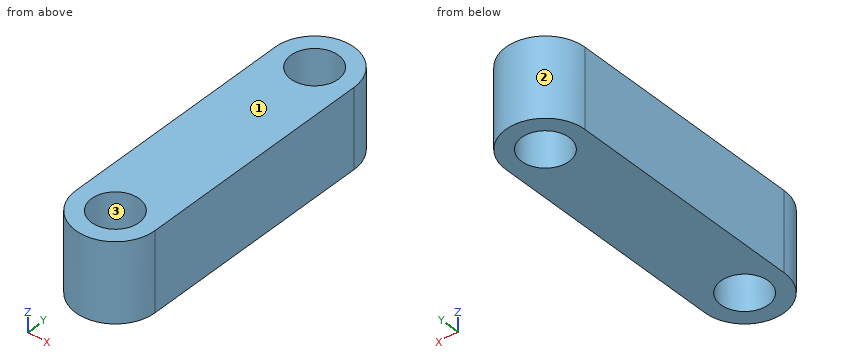
Autodesk Inventor part; units mm, degrees
ref_plane "YZ Plane" through (0, 0, 0) normal (1, 0, 0) x (0, 1, 0)
ref_plane "XZ Plane" through (0, 0, 0) normal (0, 1, 0) x (-1, 0, 0)
ref_plane "XY Plane" through (0, 0, 0) normal (0, 0, 1) x (1, 0, 0)
sketch "Sketch1" plane through (0, 0, 0) normal (0, 0, 1) x (1, 0, 0)
  circle A0 centre (0, 0) radius 1.5
  circle A1 centre (0, 0) radius 2.5
  line L0 (0, 0) -> (0, 15)
  circle A2 centre (0, 15) radius 1.5
  circle A3 centre (0, 15) radius 2.5
  line L1 (-2.5, 0) -> (-2.5, 15)
  line L2 (2.5, 0) -> (2.5, 15)
  dimension "d0" = 3
  dimension "d1" = 5
  dimension "d2" = 15
  dimension "d3" = 3
  dimension "d4" = 5
extrude "Extrusion1" add sketch "Sketch1" along normal blind 5
properties part number "bar_mid_2"
Verification items for the finished model (mm, model axes). Face numbers are marked on the shaded views. Round coordinates to 2 decimals unless told otherwise and drop trailing zeros. Order: outer loops, then holes, each group sorted by start corner. A loop starts at its lowest first (then second) coordinate and runs counter-clockwise, first axis right, second up. Notation, with made-up numbers: (52.25, 21.5) -> (80.25, 21.5) arc R21 ccw to (80.25, 58.5) -> close; hole circle Ø7 at (0.5, -1.75). An arc over 180 degrees is marked (long way). Put each result on its own line as item: value.
1) Depth check by flat-ended pin: pin 1 (1.8 mm diameter, centred on x = 0, y = 15, fed in from +Z). Enter the tip coordinate at first touch or a pass-through.
Final values:
pin 1: passes through
2) Section check C-C (y = 15.25). Record the cut outline in (x, z), then the cut area to 3 significant figures.
Final values:
outline: (-2.49, 0) -> (-1.48, 0) -> (-1.48, 5) -> (-2.49, 5) -> close; (1.48, 0) -> (2.49, 0) -> (2.49, 5) -> (1.48, 5) -> close
area: 10.1 mm^2
3) Mould release check, pull along X, two halves, no side actions. Record for the marked faces 1, 2 and 3: +X half, -X half, draft (parallel to the pull), parting line (faces both ways), or undercut.
Final values:
face 1: draft
face 2: parting line
face 3: undercut
4) Material ranges on line 1 (Y direction, x = 0, z = 2.5); line 2 (X direction, y = 15, z = 4.3); line 3 (Y direction, x = -0.8, z = 4.15), recorded low to high.
Final values:
line 1: y = -2.5 to -1.5, 1.5 to 13.5, 16.5 to 17.5
line 2: x = -2.5 to -1.5, 1.5 to 2.5
line 3: y = -2.37 to -1.27, 1.27 to 13.73, 16.27 to 17.37
5) Section check A-A (x = 0). Record the cut outline in (y, z).
Final values:
outline: (-2.5, 0) -> (-1.5, 0) -> (-1.5, 5) -> (-2.5, 5) -> close; (1.5, 0) -> (13.5, 0) -> (13.5, 5) -> (1.5, 5) -> close; (16.5, 0) -> (17.5, 0) -> (17.5, 5) -> (16.5, 5) -> close
6) Section check D-D (x = -2). Record the cut outline in (y, z).
Final values:
outline: (-1.5, 0) -> (16.5, 0) -> (16.5, 5) -> (-1.5, 5) -> close
7) Section check B-B (z = 1.55). Record the cut outline in (x, y), then the cut area to 3 significant figures.
Final values:
outline: (-2.5, 0) arc R2.5 ccw to (2.5, 0) -> (2.5, 15) arc R2.5 ccw to (-2.5, 15) -> close; hole circle Ø3 at (0, 0); hole circle Ø3 at (0, 15)
area: 80.5 mm^2
